```python
from build123d import *

# Parameters (mm, degrees)
F1_DEPTH = 127
F3_DEPTH = 127
F5_DEPTH = 304.801
F7_DEPTH = 38.1
F8_R     = 12.7
F9_DEPTH = 38.1


with BuildPart() as f1:
    # F0 (on Front) → F1 (new body)
    with BuildSketch(Plane.XZ):
        Polygon((-27.676516, -34.944516), (-27.676516, 28.555484), (-59.426516, 28.555484), (-59.426516, -73.044516), (245.373484, -73.044516), (245.373484, 28.555484), (207.273484, 28.555484), (207.273484, -34.944516), align=None)
    extrude(amount=-F1_DEPTH)

    # F2 (on face) → F3 (cut)
    with BuildSketch(Plane.XZ):
        Polygon((-40.376516, 28.555484), (-59.426516, 28.555484), (-59.426516, 9.505484), align=None)
    extrude(amount=-F3_DEPTH, mode=Mode.SUBTRACT)

    # F4 (on face) → F5 (cut, through all)
    with BuildSketch(Plane.YZ.offset(245.373484)):
        Polygon((50.8, -73.044516), (63.5, -73.044516), (76.2, -73.044516), (76.2, -56.534516), (95.25, -56.534516), (95.25, -43.834516), (76.2, -43.834516), (76.2, -34.944516), (50.8, -34.944516), (50.8, -43.834516), (31.75, -43.834516), (31.75, -56.534516), (50.8, -56.534516), align=None)
    extrude(amount=-F5_DEPTH, mode=Mode.SUBTRACT)

    # F6 (on face) → F7 (cut)
    with BuildSketch(Plane.YZ.offset(245.373484)):
        with BuildLine():
            Line((0, 28.555484), (0, -22.244516))
            Line((0, -22.244516), (15.875, -22.244516))
            Line((15.875, -22.244516), (42.406574, 17.305657))
            ThreePointArc((42.406574, 17.305657), (51.547059, 25.567249), (63.5, 28.555484))
            Line((63.5, 28.555484), (0, 28.555484))
        make_face()
        with BuildLine():
            Line((127, 28.555484), (63.5, 28.555484))
            ThreePointArc((63.5, 28.555484), (75.452941, 25.567249), (84.593426, 17.305657))
            Line((84.593426, 17.305657), (111.125, -22.244516))
            Line((111.125, -22.244516), (127, -22.244516))
            Line((127, -22.244516), (127, 28.555484))
        make_face()
    extrude(amount=-F7_DEPTH, mode=Mode.SUBTRACT)

    # F8 (on face) → F9 (cut)
    with BuildSketch(Plane.YZ.offset(245.373484)):
        with Locations((63.5, 3.155484)):
            Circle(F8_R)
    extrude(amount=-F9_DEPTH, mode=Mode.SUBTRACT)


solid = f1.part
```
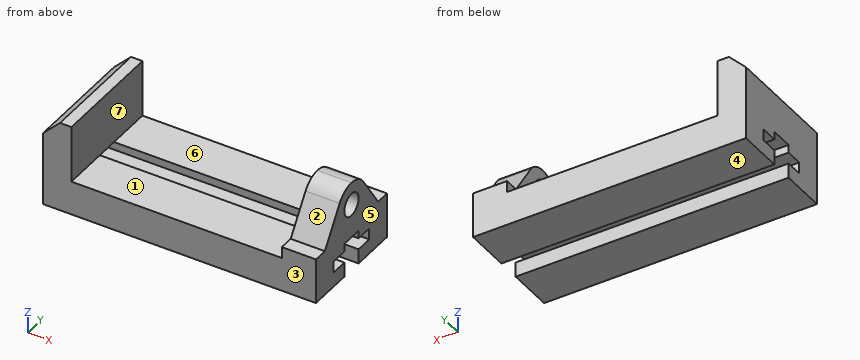
For this review, take the finished solid that the model builds, in its own axes (mm). Face numbers are marked on the shaded views. A direction names the side the tool comes from. Give positions to 0.01 mm unless a question says otherwise; leave off trailing zeros. Write each loop counter-clockwise with the first axis right and the second up, starting at its lowest first coordinate (ties: lowest second). Pieces come first, ordered by that corner, then holes. Notation, with made-up numbers: M 79.5,-37.5 L 114.5,-37.5 A8 ccw 114.5,-33.5 Z; hole C -8,57.25 d4. An arc over 180 degrees is marked long. One line per item, written item: value.
1) Take a section at D-D, the plane x = -35.5. Write out the cut boundary in (y, z).
Results are:
outline: M 0,-73.04 L 50.8,-73.04 L 50.8,-56.53 L 31.75,-56.53 L 31.75,-43.83 L 50.8,-43.83 L 50.8,-34.94 L 76.2,-34.94 L 76.2,-43.83 L 95.25,-43.83 L 95.25,-56.53 L 76.2,-56.53 L 76.2,-73.04 L 127,-73.04 L 127,28.56 L 0,28.56 Z
2) The part is to be moulded in two halves that separate along X. For the marked faces 4, 5, 6 and 7, say which applies: +X half, -X half, draft (parallel to the pull), parting line (faces both ways), or undercut.
Results are:
face 4: draft
face 5: +X half
face 6: undercut
face 7: undercut
3) For line 1 (Z direction, x = 232.5, y = 63.5); line 2 (Y direction, x = 0, z = -39.5); line 3 (Y direction, x = 124.5, z = -52.5), list the stretches that pass through material, from the lowest coordinate up. Write a range as from..to.
Results are:
line 1: z = -34.94..-9.54, 15.86..28.56
line 2: y = 0..50.8, 76.2..127
line 3: y = 0..31.75, 95.25..127
4) For the marked faces 1, 2 and 3, list the 3-axis set-ups (+Z, -Z, +X, -X, +Y, -Y) from which the entire face can be reached by the end or side of a thin tool; tool diameter is ignored.
Results are:
face 1: +Z, +Y, -Y
face 2: +Z, +X, -Y
face 3: +Z, -Z, +X, -X, -Y
5) For P1, Ø15, axis at x = 83.5, y = 42.5, coming from the +Z side; P2, Ø20.5, axis at x = -49.5, y = 63, coming from the -Z side; P3, Ø19, axis at y = 47.5, z = 11.5, coming from the -X side; P4, Ø5, axis at x = 219, y = 11.5, coming from the +Z side, all flat-tipped, find the tip position at first contact; note any pin that passes through.
Results are:
P1: stops at z = -34.94
P2: stops at z = -34.94
P3: stops at x = -59.43
P4: stops at z = -22.24
6) Take a section at B-B, the plane y = 115. Write out the cut boundary in (x, z).
Results are:
outline: M -59.43,-73.04 L 245.37,-73.04 L 245.37,-22.24 L 207.27,-22.24 L 207.27,-34.94 L -27.68,-34.94 L -27.68,28.56 L -40.38,28.56 L -59.43,9.51 Z
7) Take a section at C-C, the plane z = -1.5. Write out the cut boundary in (x, y).
Results are:
outline: M -59.43,0 L -27.68,0 L -27.68,127 L -59.43,127 Z; M 207.27,29.79 L 245.37,29.79 L 245.37,51.68 L 207.27,51.68 Z; M 207.27,75.32 L 245.37,75.32 L 245.37,97.21 L 207.27,97.21 Z
8) Take a section at A-A, the plane x = 188.5. Write out the cut boundary in (y, z), then the cut area to 3 significant figures.
Results are:
outline: M 0,-73.04 L 50.8,-73.04 L 50.8,-56.53 L 31.75,-56.53 L 31.75,-43.83 L 50.8,-43.83 L 50.8,-34.94 L 0,-34.94 Z; M 76.2,-73.04 L 127,-73.04 L 127,-34.94 L 76.2,-34.94 L 76.2,-43.83 L 95.25,-43.83 L 95.25,-56.53 L 76.2,-56.53 Z
area: 3,390 mm²
